Part model, mm, in its own coordinate system. Face numbers are marked on the shaded views. A direction names the side the tool comes from. Give positions to 0.01 mm unless a question says otherwise; leave off trailing zeros. Order: outer loops, then holes, each group sorted by start corner. A loop starts at its lowest first (then second) coordinate and runs counter-clockwise, first axis right, second up.
1. Slice it at A-A on z = 3.8. List the corners of the cut face in (x, y), and give its area (3 significant figures).
2. Slice it at B-B on y = 11.75. List the corners of the cut face in (x, z).
3. Mould opens along X. For the marked faces 3, 4 and 5 say: +X half, -X half, draft (parallel to the pull), parting line (faces both ways), or undercut.
4. Drop a flat-ended pin along its axis: pin 1 Ø6.5 at (x, y) = (10.5, 8) entering from +Z. Give the stop position or say it passes through.
5. Probe line 1 (X direction, y = 2.25, z = 2.4); line 2 (Y direction, x = 14, z = 4.75); line 3 (Z direction, x = 13, y = 6). List the from-to ranges inside material, lowest first.
6. Slice it at C-C on x = 9. List the corners of the cut face in (y, z), and give its area (3 significant figures).
7. Which spindle directions (+Z, -Z, +X, -X, +Y, -Y) get a long thin tool onto all of the face, cutting with end or side? Do the marked faces 1 and 2. Say none if no direction does.
Autodesk Inventor part; units mm, degrees
ref_plane "YZ Plane" through (0, 0, 0) normal (1, 0, 0) x (0, 1, 0)
ref_plane "XZ Plane" through (0, 0, 0) normal (0, 1, 0) x (-1, 0, 0)
ref_plane "XY Plane" through (0, 0, 0) normal (0, 0, 1) x (1, 0, 0)
sketch "Sketch1" plane through (0, 0, 0) normal (0, 0, 1) x (1, 0, 0)
  line L0 (0, 13.3457) -> (19.68, 13.3457)
  line L1 (19.68, 13.3457) -> (19.68, -0.5024)
  line L2 (19.68, -0.5024) -> (0, -0.5024)
  line L3 (0, -0.5024) -> (0, 13.3457)
  point P0 (0, 0)
extrude "Extrusion1" add sketch "Sketch1" along normal blind 5.0038
shell "Shell1" thickness 0.6 removed faces 1 at (6.56, 4.1137, 5.0038)
sketch "Sketch2" plane through (19.08, 0.0976, 0.6) normal (-1, 0, 0) x (0, 0, 1)
  point P0 (-0.6, -0.0976)
  point P1 (2.0364, 9.2348)
hole "Hole1" at (19.08, 9.3324, 2.6364) direction (1, 0, 0) diameter 0.762 end through all
properties part number "a1"
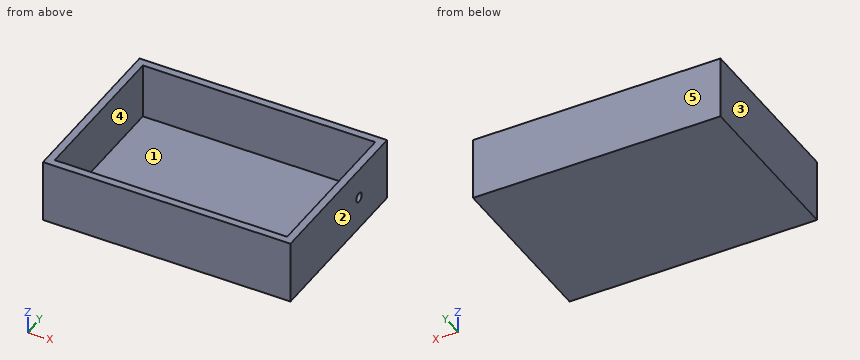
Data:
1. outline: (0, -0.5) - (19.68, -0.5) - (19.68, 13.35) - (0, 13.35) - close; hole (0.6, 0.1) - (19.08, 0.1) - (19.08, 12.75) - (0.6, 12.75) - close
1. area: 38.8 mm2
2. outline: (0, 0) - (19.68, 0) - (19.68, 5) - (19.08, 5) - (19.08, 0.6) - (0.6, 0.6) - (0.6, 5) - (0, 5) - close
3. face 3: -X half
3. face 4: undercut
3. face 5: draft
4. pin 1: stops at z = 0.6
5. line 1: x = 0 to 0.6, 19.08 to 19.68
5. line 2: y = -0.5 to 0.1, 12.75 to 13.35
5. line 3: z = 0 to 0.6
6. outline: (-0.5, 0) - (13.35, 0) - (13.35, 5) - (12.75, 5) - (12.75, 0.6) - (0.1, 0.6) - (0.1, 5) - (-0.5, 5) - close
6. area: 13.6 mm2
7. face 1: +Z
7. face 2: +Z, -Z, +X, +Y, -Y
